from build123d import *

# Parameters (mm, degrees)
BOX720_W               = 80
BOX720_H               = 6
BOX720_DEPTH           = 20
BOX720_PLACEMENT_ANGLE = 71
BOX727_W               = 44
BOX727_H               = 6
BOX727_DEPTH           = 49


with BuildPart() as krychle720:
    # Box720 → Box720 (new body)
    with BuildSketch(Plane.XY):
        with Locations((40, 3)):
            Rectangle(BOX720_W, BOX720_H)
    extrude(amount=BOX720_DEPTH)


with BuildPart() as krychle720_1:
    # Box720 placement: moved
    add(krychle720.part.moved(Location((-118.17, -24, 82.63))).rotate(Axis((-118.17, -24, 82.63), (0, 1, 0)), BOX720_PLACEMENT_ANGLE))


with BuildPart() as cut532:
    # Box727 → Box727 (new body)
    with BuildSketch(Plane(origin=(-93, -24, 29), x_dir=(1, 0, 0), z_dir=(0, 0, 1))):
        with Locations((22, 3)):
            Rectangle(BOX727_W, BOX727_H)
    extrude(amount=BOX727_DEPTH)

    # Cut532: cut Krychle720
    add(krychle720_1.part, mode=Mode.SUBTRACT)


solid = cut532.part
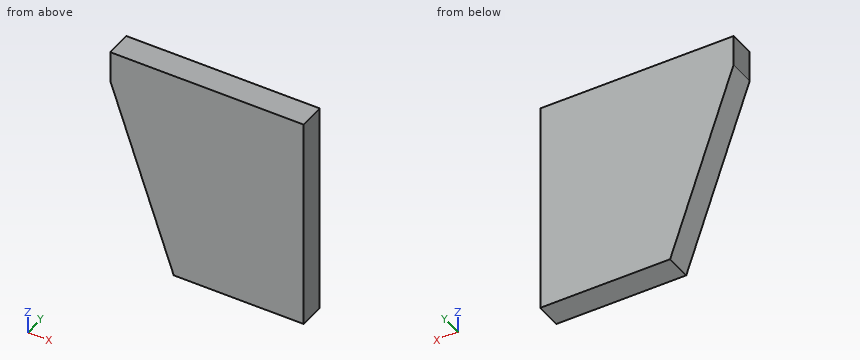
For this review, take the finished solid that the model builds, in its own axes (mm). Give positions to 0.01 mm unless a question says otherwise; leave off trailing zeros. Order: outer loops, then holes, each group sorted by start corner. A loop starts at its lowest first (then second) coordinate and runs counter-clockwise, first axis right, second up. Notation, with made-up numbers: M -25,70.5 L 26,70.5 A19 cw 26,96.5 Z; hole C 68.25,1.25 d1. An arc over 180 degrees is marked long. Answer in a Markdown table with one row per item. Add a question column.
(1) Consider section B-B on z = 45. State the section outline as (x, y) points.
(2) Consider section A-A on y = -18.85. State the section outline as (x, z) points.
(3) Consider section C-C on z = 55.5. State the section outline as (x, y) points.
(4) Wall thickness on probe 1 along X at (y, z) = (-20, 34); probe 2 along X at (y, z) = (-19.1, 56.5): over which ranges is each line inside the solid? List them lowest first. Write a range as [from, to].
Evaluation:
| question | item | result |
|---|---|---|
| 1 | outline | M -84.06,-24 L -49,-24 L -49,-18 L -84.06,-18 Z |
| 2 | outline | M -93,70.96 L -78.55,29 L -49,29 L -49,78 L -93,78 Z |
| 3 | outline | M -87.68,-24 L -49,-24 L -49,-18 L -87.68,-18 Z |
| 4 | probe 1 | x = [-80.27, -49] |
| 4 | probe 2 | x = [-88.02, -49] |
